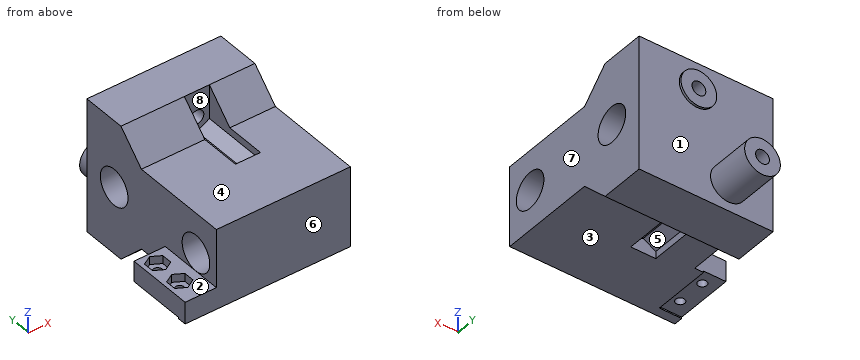
from build123d import *

# Parameters (mm, degrees)
SKETCH_1_W           = 30
SKETCH_1_H           = 30
EXTRUDE_1_DEPTH      = 38
SKETCH_3_R           = 4
EXTRUDE_3_DEPTH      = 10
SKETCH_7_R           = 4
EXTRUDE_4_DEPTH      = 0.5
SKETCH_6_R           = 4.05
CUT_EXTRUDE_3_DEPTH  = 31
SKETCH_9_R           = 1.55
CUT_EXTRUDE_4_DEPTH  = 21
CUT_EXTRUDE_6_DEPTH  = 31
CUT_EXTRUDE_5_DEPTH  = 15
SKETCH_12_W          = 4.9
SKETCH_12_H          = 15
EXTRUDE_5_DEPTH      = 7
SKETCH_14_W          = 0.3
SKETCH_14_H          = 13
CUT_EXTRUDE_7_DEPTH  = 5
SKETCH_15_R          = 1
CUT_EXTRUDE_8_DEPTH  = 24.7
CUT_EXTRUDE_10_DEPTH = 1.8


with BuildPart() as part:
    # 草图1 → 凸台-拉伸1 (new body)
    with BuildSketch(Plane(origin=(0, 0, 0), x_dir=(1, 0, 0), z_dir=(0, 1, 0))):
        with Locations((15, 15)):
            Rectangle(SKETCH_1_W, SKETCH_1_H)
    extrude(amount=EXTRUDE_1_DEPTH)

    # 草图3 → 凸台-拉伸3 (add)
    with BuildSketch(Plane(origin=(0, 38, -50), x_dir=(1, 0, 0), z_dir=(0, -1, 0))):
        with Locations((10, 26)):
            Circle(SKETCH_3_R)
    extrude(amount=-EXTRUDE_3_DEPTH)

    # 草图7 → 凸台-拉伸4 (add)
    with BuildSketch(Plane.XZ.offset(-38)):
        with Locations((17, -6)):
            Circle(SKETCH_7_R)
    extrude(amount=-EXTRUDE_4_DEPTH)

    # 草图6 → 切除-拉伸3 (cut, through all)
    with BuildSketch(Plane(origin=(30, 0, 0), x_dir=(0, 0, -1), z_dir=(1, 0, 0))):
        with Locations((15, 6)):
            Circle(SKETCH_6_R)
        with Locations((15, 30)):
            Circle(SKETCH_6_R)
    extrude(amount=-CUT_EXTRUDE_3_DEPTH, mode=Mode.SUBTRACT)

    # 草图9 → 切除-拉伸4 (cut, through all)
    with BuildSketch(Plane(origin=(0, 28, 0), x_dir=(1, 0, 0), z_dir=(0, 1, 0))):
        with Locations((17, 6)):
            Circle(SKETCH_9_R)
        with Locations((10, 24)):
            Circle(SKETCH_9_R)
    extrude(amount=CUT_EXTRUDE_4_DEPTH, mode=Mode.SUBTRACT)

    # 草图11 → 切除-拉伸6 (cut, through all)
    with BuildSketch(Plane(origin=(30, 0, 0), x_dir=(0, 0, -1), z_dir=(1, 0, 0))):
        Polygon((6, 0), (6, 22), (0, 28), (0, 0), align=None)
        Polygon((24, 0), (24, 22), (30, 28), (30, 0), align=None)
    extrude(amount=-CUT_EXTRUDE_6_DEPTH, mode=Mode.SUBTRACT)

    # 草图10 → 切除-拉伸5 (cut)
    with BuildSketch(Plane(origin=(0, 28, 0), x_dir=(1, 0, 0), z_dir=(0, 1, 0))):
        Polygon((19.8, 0), (19.8, 7.616580754), (17, 9.233161507), (14.2, 7.616580754), (14.2, 0), align=None)
        Polygon((10, 20.766838493), (12.8, 22.383419246), (12.8, 30), (7.2, 30), (7.2, 22.383419246), align=None)
    extrude(amount=-CUT_EXTRUDE_5_DEPTH, mode=Mode.SUBTRACT)

    # 草图12 → 凸台-拉伸5 (add)
    with BuildSketch(Plane.ZY):
        with Locations((-21.55, 7.5)):
            Rectangle(SKETCH_12_W, SKETCH_12_H)
    extrude(amount=EXTRUDE_5_DEPTH)

    # 草图14 → 切除-拉伸7 (cut)
    with BuildSketch(Plane.ZY.offset(7)):
        with Locations((-23.85, 8.5)):
            Rectangle(SKETCH_14_W, SKETCH_14_H)
    extrude(amount=-CUT_EXTRUDE_7_DEPTH, mode=Mode.SUBTRACT)

    # 草图15 → 切除-拉伸8 (cut, through all)
    with BuildSketch(Plane(origin=(0, 0, -23.7), x_dir=(-1, 0, 0), z_dir=(0, 0, -1))):
        with Locations((4, 12)):
            Circle(SKETCH_15_R)
        with Locations((4, 5.5)):
            Circle(SKETCH_15_R)
    extrude(amount=-CUT_EXTRUDE_8_DEPTH, mode=Mode.SUBTRACT)

    # 草图17 → 切除-拉伸10 (cut)
    with BuildSketch(Plane.XY.offset(-19.1)):
        Polygon((-1.95, 10.816431948), (-1.95, 13.183568052), (-4, 14.367136104), (-6.05, 13.183568052), (-6.05, 10.816431948), (-4, 9.632863896), align=None)
        Polygon((-1.95, 4.316431948), (-1.95, 6.683568052), (-4, 7.867136104), (-6.05, 6.683568052), (-6.05, 4.316431948), (-4, 3.132863896), align=None)
    extrude(amount=-CUT_EXTRUDE_10_DEPTH, mode=Mode.SUBTRACT)


solid = part.part
Source: CAD feature listing. Evaluate the final solid. Frame: model axes, mm. Face numbers are marked on the shaded views. A direction names the side the tool comes from. Coordinates: 2 decimals unless noted, no trailing zeros. Loops run counter-clockwise (first coordinate to the right, second up) from the corner with the lowest first, then second, coordinate; pieces in that order, holes last. Notation, with made-up numbers: (-14, 25) -> (36, 25) arc R12 ccw to (36, 29) -> close; hole circle Ø3 at (-33.75, 74.25). An arc over 180 degrees is marked (long way). Answer in a Markdown table with one row per item. Add a question column.
Q1. Section B-B on x = 1.5. Return the cut outline in (y, z).
Q2. Section D-D on y = 35. Return the cut outline in (x, z).
Q3. Contact query for flat-ended pins moving along their axis: pin 1 Ø4.5 at (x, y) = (-4, 11) entering from +Z; pin 2 Ø10 at (x, z) = (-2, -22) entering from -Y; pin 3 Ø4 at (x, y) = (-1.5, 18) entering from -Z; pin 4 Ø1.5 at (y, z) = (22, -11.5) entering from -X. Output: stop coordinate, or through.
Q4. Pull-direction query (X, two-part tool) for the marked faces 6, 7 and 8; classes: pulls with the +X half, pulls with the -X half, needs draft (parallel to the pull), parting line crosses it, or undercut.
Q5. Section C-C on z = -15. Return the cut outline in (x, y).
Q6. Section A-A on x = 9. Return the cut outline in (y, z), and give its area (3 significant figures).
Q7. Ray query, line 1 along Y through (x, z) = (-4, -22); line 2 along Y through (x, z) = (18.25, -15); line 3 along X through (y, z) = (32, -24). Return the intervals inside material, ascending.
Q8. Reachability of the marked faces 1, 2, 3, 4 and 5 from +Z, -Z, +X, -X, +Y, -Y: full face, straight path, thin tool, end or side. Return the list, or none.
Computed values:
| question | item | result |
|---|---|---|
| 1 | outline | (0, -24) -> (22, -24) -> (28, -30) -> (38, -30) -> (38, 0) -> (28, 0) -> (22, -6) -> (0, -6) -> close; hole circle Ø8.1 at (6, -15); hole circle Ø8.1 at (30, -15) |
| 2 | outline | (0, -30) -> (30, -30) -> (30, 0) -> (0, 0) -> close; hole circle Ø3.1 at (10, -24); hole circle Ø3.1 at (17, -6) |
| 3 | pin 1 | stops at z = -19.1 |
| 3 | pin 2 | stops at y = 0 |
| 3 | pin 3 | stops at z = -24 |
| 3 | pin 4 | stops at x = 0 |
| 4 | face 6 | needs draft |
| 4 | face 7 | pulls with the +X half |
| 4 | face 8 | undercut |
| 5 | outline | (0, 0) -> (30, 0) -> (30, 1.95) -> (0, 1.95) -> close; (0, 10.05) -> (30, 10.05) -> (30, 25.95) -> (0, 25.95) -> close; (0, 34.05) -> (30, 34.05) -> (30, 38) -> (0, 38) -> close |
| 6 | outline | (0, -24) -> (13, -24) -> (13, -21.34) -> (28, -21.34) -> (28, -22.82) -> (48, -22.82) -> (48, -20.13) -> (38, -20.13) -> (38, 0) -> (28, 0) -> (22, -6) -> (0, -6) -> close; (28, -30) -> (38, -30) -> (38, -27.87) -> (48, -27.87) -> (48, -25.18) -> (28, -25.18) -> close; hole circle Ø8.1 at (6, -15); hole circle Ø8.1 at (30, -15) |
| 6 | area | 709 mm^2 |
| 7 | line 1 | y = 0 to 4.5, 6.5 to 11, 13 to 15 |
| 7 | line 2 | y = 0 to 1.95, 10.05 to 25.95, 34.05 to 38 |
| 7 | line 3 | x = 0 to 8.45, 11.55 to 30 |
| 8 | face 1 | +Y |
| 8 | face 2 | +Z, -X, +Y, -Y |
| 8 | face 3 | -Z, +X, -X, -Y |
| 8 | face 4 | +Z, +X, -X, -Y |
| 8 | face 5 | -Z |
